Part model, mm, in its own coordinate system. Face numbers are marked on the shaded views. A direction names the side the tool comes from. Round coordinates to 2 decimals unless told otherwise and drop trailing zeros. Loops run counter-clockwise (first coordinate to the right, second up) from the corner with the lowest first, then second, coordinate; pieces in that order, holes last.
(1) Cut at A-A on x = 0. List the corners of the cut face in (y, z).
(2) Tool access for the marked faces 1, 2 and 3: list every direction of +Z, -Z, +X, -X, +Y, -Y with a clear straight run to the whole face (end or side of a thin tool).
(3) Flat gauge pins, fed straight in: pin 1 (1.4 mm diameter, centred on y = 4, z = 1.5, fed in from -X); pin 2 (3 mm diameter, centred on x = -3, y = 0, fed in from -Z); pin 3 (1.3 mm diameter, centred on y = 8, z = -1, fed in from -X); pin 4 (0.6 mm diameter, centred on x = 0, z = 1.5, fed in from -Y). Where does each tip first touch, or does it go through?
(4) Cut at C-C on y = 7.5. Count the separate pieces of the cut face and the enclosed holes in it, then the cut area to 3 significant figures.
(5) Cut at D-D on z = 1.7. List the corners of the cut face in (x, y), then the cut area to 3 significant figures.
(6) Probe probe 1 along X at (y, z) = (4, 0.05); probe 2 along Z at (x, y) = (-0.75, 4.75); probe 3 along X at (y, z) = (0, 0.85). List the from-to ranges inside material, lowest first.
(7) Cut at B-B on y = 0. List the corners of the cut face in (x, z).
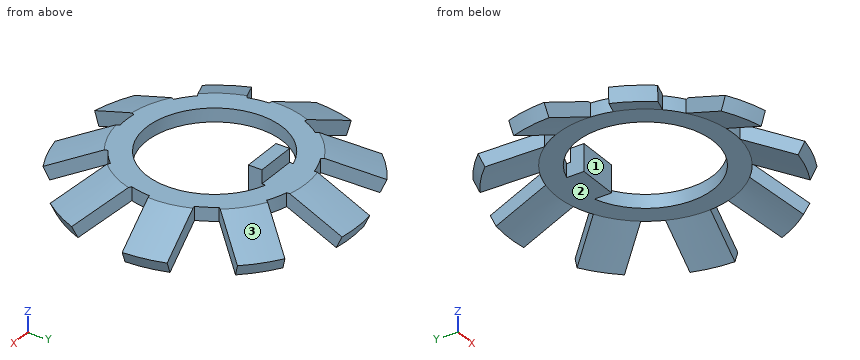
from build123d import *

# Parameters (mm, degrees)
CUT_EXTRUDE1_DEPTH  = 15.942649011
CIRPATTERN1_START   = -1.668160675
CIRPATTERN1_DEPTH   = 2.668160675
BOSS_EXTRUDE1_DEPTH = 1.5


# Read off the part's stored shape, not the designer's step: CirPattern1
with BuildPart() as part:
    # Sketch1 → Revolve1 (revolve)
    with BuildSketch(Plane(origin=(0, 0, 0), x_dir=(0, 0, -1), z_dir=(1, 0, 0)), mode=Mode.PRIVATE) as revolve1_sk:
        Polygon((0.761852714, 10.5), (-1, 6.721694663), (-1, 5), (0, 5), (0, 6.5), (1.668160501, 10.077381738), align=None)
    revolve(revolve1_sk.sketch.rotate(Axis((0, 0, 0), (0, 0, 1)), 90), axis=Axis((0, 0, 0), (0, 0, 1)))

    # Sketch2 → Cut-Extrude1 (cut, symmetric)
    with BuildSketch(Plane.XY):
        with BuildLine():
            Line((1.5, 10.392304845), (1.5, 6.32455532))
            ThreePointArc((1.5, 6.32455532), (2.223130932, 6.108002035), (2.916279132, 5.809071873))
            Line((2.916279132, 5.809071873), (5.530978126, 8.925148793))
            ThreePointArc((5.530978126, 8.925148793), (3.591211505, 9.866772518), (1.5, 10.392304845))
        make_face()
    extrude(amount=CUT_EXTRUDE1_DEPTH, both=True, mode=Mode.SUBTRACT)

    # CirPattern1 outline → CirPattern1 (cut)
    with BuildSketch(Plane.XY.offset(CIRPATTERN1_START)):
        with BuildLine():
            ThreePointArc((-2.916279132, 5.809071873), (-2.223130932, 6.108002035), (-1.5, 6.32455532))
            Line((-1.5, 6.32455532), (-1.5, 12))
            Line((-1.5, 12), (-8.111084639, 12))
            Line((-8.111084639, 12), (-5.530978126, 8.925148793))
            Line((-5.530978126, 8.925148793), (-2.916279132, 5.809071873))
        make_face()
        with BuildLine():
            Line((12, 3.639063687), (12, 11.96745737))
            Line((12, 11.96745737), (7.829111455, 6.996785963))
            Line((7.829111455, 6.996785963), (5.214412461, 3.880709044))
            ThreePointArc((5.214412461, 3.880709044), (5.629165125, 3.25), (5.967998847, 2.575459135))
            Line((5.967998847, 2.575459135), (9.973950117, 3.281816428))
            Line((9.973950117, 3.281816428), (12, 3.639063687))
        make_face()
        with BuildLine():
            Line((-7.829111455, 6.996785963), (-12, 11.96745737))
            Line((-12, 11.96745737), (-12, 3.639063687))
            Line((-12, 3.639063687), (-9.973950117, 3.281816428))
            Line((-9.973950117, 3.281816428), (-5.967998847, 2.575459135))
            ThreePointArc((-5.967998847, 2.575459135), (-5.629165125, 3.25), (-5.214412461, 3.880709044))
            Line((-5.214412461, 3.880709044), (-7.829111455, 6.996785963))
        make_face()
        with BuildLine():
            Line((12, -5.196152423), (12, 0.592783851))
            Line((12, 0.592783851), (10.49489465, 0.327393169))
            Line((10.49489465, 0.327393169), (6.48894338, -0.378964124))
            ThreePointArc((6.48894338, -0.378964124), (6.401250395, -1.128713155), (6.227225575, -1.863239554))
            Line((6.227225575, -1.863239554), (9.75, -3.897114317))
            Line((9.75, -3.897114317), (12, -5.196152423))
        make_face()
        with BuildLine():
            Line((-10.49489465, 0.327393169), (-12, 0.592783851))
            Line((-12, 0.592783851), (-12, -5.196152423))
            Line((-12, -5.196152423), (-9.75, -3.897114317))
            Line((-9.75, -3.897114317), (-6.227225575, -1.863239554))
            ThreePointArc((-6.227225575, -1.863239554), (-6.401250395, -1.128713155), (-6.48894338, -0.378964124))
            Line((-6.48894338, -0.378964124), (-10.49489465, 0.327393169))
        make_face()
        with BuildLine():
            Line((12, -12), (12, -8.660254037))
            Line((12, -8.660254037), (8.25, -6.495190528))
            Line((8.25, -6.495190528), (4.727225575, -4.461315766))
            ThreePointArc((4.727225575, -4.461315766), (4.178119463, -4.97928888), (3.572664248, -5.430107749))
            Line((3.572664248, -5.430107749), (4.963916524, -9.252541961))
            Line((4.963916524, -9.252541961), (5.96390947, -12))
            Line((5.96390947, -12), (12, -12))
        make_face()
        with BuildLine():
            Line((-8.25, -6.495190528), (-12, -8.660254037))
            Line((-12, -8.660254037), (-12, -12))
            Line((-12, -12), (-5.96390947, -12))
            Line((-5.96390947, -12), (-4.963916524, -9.252541961))
            Line((-4.963916524, -9.252541961), (-3.572664248, -5.430107749))
            ThreePointArc((-3.572664248, -5.430107749), (-4.178119463, -4.97928888), (-4.727225575, -4.461315766))
            Line((-4.727225575, -4.461315766), (-8.25, -6.495190528))
        make_face()
        with BuildLine():
            Line((-2.771376153, -12), (2.771376153, -12))
            Line((2.771376153, -12), (2.144838662, -10.278602391))
            Line((2.144838662, -10.278602391), (0.753586386, -6.456168179))
            ThreePointArc((0.753586386, -6.456168179), (0, -6.5), (-0.753586386, -6.456168179))
            Line((-0.753586386, -6.456168179), (-2.144838662, -10.278602391))
            Line((-2.144838662, -10.278602391), (-2.771376153, -12))
        make_face()
    extrude(amount=CIRPATTERN1_DEPTH, mode=Mode.SUBTRACT)

    # Sketch3 → Boss-Extrude1 (add, symmetric)
    with BuildSketch(Plane(origin=(0, 0, 0), x_dir=(0, 0, -1), z_dir=(1, 0, 0))):
        Polygon((-2, 4.5), (-1, 4.5), (-1, 5), (0, 5), (0, 3.5), (-2, 3.5), align=None)
    extrude(amount=BOSS_EXTRUDE1_DEPTH, both=True)


solid = part.part
Final values:
1. outline: (-6.5, 0) - (-5, 0) - (-5, 1) - (-6.5, 1) - close; (3.5, 0) - (6.5, 0) - (10.08, -1.67) - (10.5, -0.76) - (6.72, 1) - (4.5, 1) - (4.5, 2) - (3.5, 2) - close
2. face 1: +Z, -Z
2. face 2: -Z
2. face 3: +Z, +X, +Y
3. pin 1: stops at x = -5.56
3. pin 2: passes through
3. pin 3: stops at x = -7.45
3. pin 4: stops at y = 3.5
4. separate pieces: 3
4. enclosed holes: 0
4. area: 9.28 mm2
5. outline: (-1.5, 3.5) - (1.5, 3.5) - (1.5, 4.5) - (-1.5, 4.5) - close
5. area: 3.00 mm2
6. probe 1: x = -5.31 to -3, -1.5 to 1.5, 3 to 5.31
6. probe 2: z = 0 to 1
6. probe 3: x = -7.04 to -5, 5 to 7.04
7. outline: (-8.64, -1) - (-6.5, 0) - (-5, 0) - (-5, 1) - (-6.72, 1) - (-8.64, 0.11) - close; (5, 0) - (6.5, 0) - (8.64, -1) - (8.64, 0.11) - (6.72, 1) - (5, 1) - close
